Print and shaded views of the part. All mm, measured from the part's lowest x, y and z. Round coordinates to 2 decimals unless told otherwise and drop trailing zeros. Write each loop counter-clockwise with the first axis right and the second up, starting at its lowest first coordinate (ties: lowest second). Pieces come first, ordered by that corner, then holes. Notation, with made-up numbers: (-10, -14) - (14, -14) arc R26 cw to (14, 12) - close; hole circle Ø10 at (1, 53.5). An arc over 180 degrees is marked (long way). One line per item, written item: value.
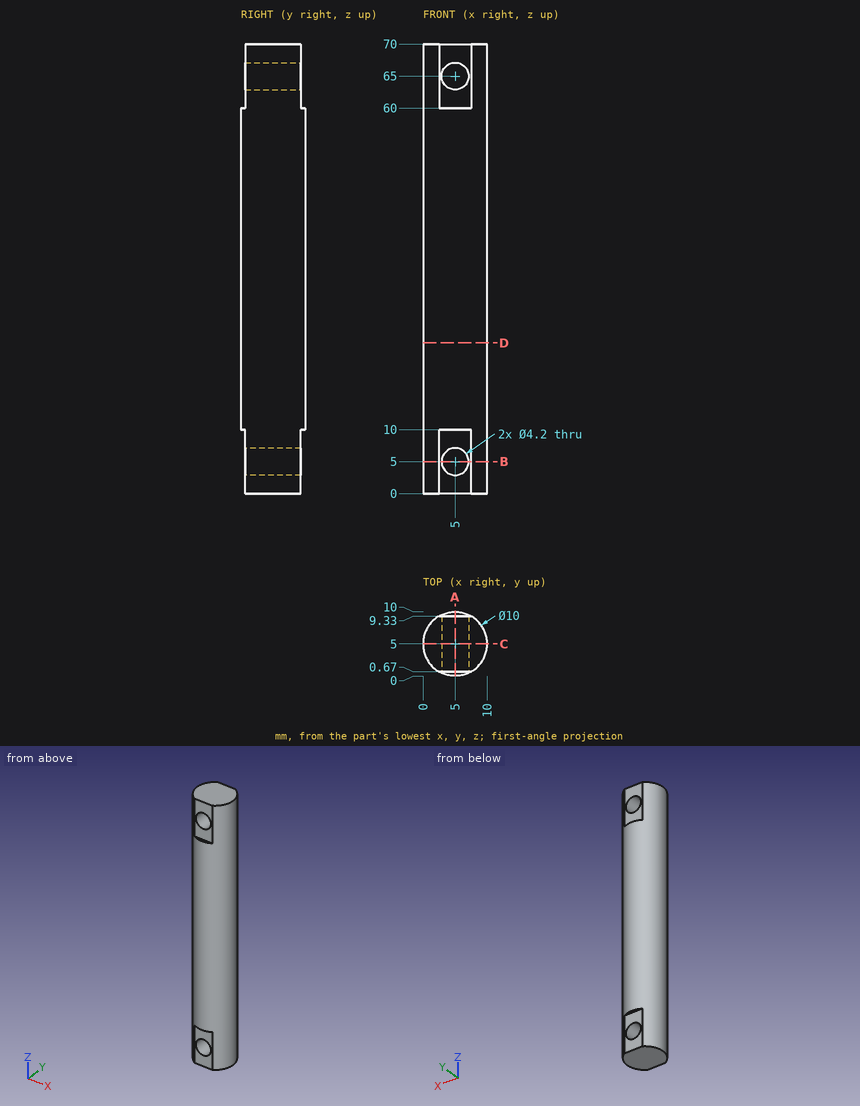
1. Band-saw the part on D-D on z = 23.5. Write the cut outline in (x, y).
Report:
outline: circle Ø10 at (5, 5)
2. Drop flat-ended pins along their axis: pin 1 (2.5 mm diameter, centred on x = 5.5, z = 4, fed in from -Y); pin 2 (2.5 mm diameter, centred on x = 5, z = 65, fed in from +Y); pin 3 (4 mm diameter, centred on y = 6.5, z = 38, fed in from -X); pin 4 (1.5 mm diameter, centred on x = 5.5, z = 66.5, fed in from +Y). Give the stop position or say it passes through.
Report:
pin 1: y = 0.67
pin 2: through
pin 3: x = 0
pin 4: y = 9.33
3. Band-saw the part on A-A on x = 5. Write the cut outline in (y, z).
Report:
outline: (0, 10) - (0.67, 10) - (0.67, 7.1) - (9.33, 7.1) - (9.33, 10) - (10, 10) - (10, 60) - (9.33, 60) - (9.33, 62.9) - (0.67, 62.9) - (0.67, 60) - (0, 60) - close; (0.67, 0) - (9.33, 0) - (9.33, 2.9) - (0.67, 2.9) - close; (0.67, 67.1) - (9.33, 67.1) - (9.33, 70) - (0.67, 70) - close
4. Band-saw the part on B-B on z = 5. Write the cut outline in (x, y), plus the area to 3 significant figures.
Report:
outline: (2.5, 0.67) - (2.9, 0.67) - (2.9, 9.33) - (2.5, 9.33) arc R5 ccw to start; (7.1, 0.67) - (7.5, 0.67) arc R5 ccw to (7.5, 9.33) - (7.1, 9.33) - close
area: 37.6 mm²
5. Band-saw the part on C-C on y = 5. Write the cut outline in (x, z).
Report:
outline: (0, 0) - (10, 0) - (10, 70) - (0, 70) - close; hole circle Ø4.2 at (5, 5); hole circle Ø4.2 at (5, 65)
6. Wall check: probe 1 along Z at (x, y) = (5.25, 7) (3 decimals); probe 2 along Z at (x, y) = (4.25, 5); probe 3 along Y at (x, z) = (7.25, 4). Give the ranges that are in metal, low to high. Write a range as [from, to].
Report:
probe 1: [0, 2.915], [7.085, 62.915], [67.085, 70]
probe 2: [0, 3.04], [6.96, 63.04], [66.96, 70]
probe 3: [0.67, 9.33]
